Build history of the part. All positions in model axes, mm. Round coordinates to 2 decimals unless told otherwise and drop trailing zeros. Order: outer loops, then holes, each group sorted by start corner. A loop starts at its lowest first (then second) coordinate and runs counter-clockwise, first axis right, second up. Notation, with made-up numbers: M -36,-3 L -31,-3 A21 ccw -31,15 Z; hole C 11.25,-18.5 d6. An arc over 180 degrees is marked long. Use CSV: the item, a comma, the result in double quotes.
from build123d import *

# Parameters (mm, degrees)
SKETCH1_W           = 100
SKETCH1_H           = 120
BOSS_EXTRUDE1_DEPTH = 1.5
SKETCH2_R           = 2.5
CUT_EXTRUDE1_DEPTH  = 1.5
SKETCH4_R           = 2.65
CUT_EXTRUDE2_DEPTH  = 1.5


with BuildPart() as part:
    # Sketch1 → Boss-Extrude1 (new body)
    with BuildSketch(Plane.XY):
        with Locations((50, 60)):
            Rectangle(SKETCH1_W, SKETCH1_H)
    extrude(amount=BOSS_EXTRUDE1_DEPTH)

    # Sketch2 → Cut-Extrude1 (cut)
    with BuildSketch(Plane(origin=(0, 0, 0), x_dir=(-1, 0, 0), z_dir=(0, 0, -1))):
        with Locations((-82.275, 20)):
            Circle(SKETCH2_R)
        with Locations((-17.725, 20)):
            Circle(SKETCH2_R)
        with Locations((-17.725, 100)):
            Circle(SKETCH2_R)
        with Locations((-82.275, 100)):
            Circle(SKETCH2_R)
    extrude(amount=-CUT_EXTRUDE1_DEPTH, mode=Mode.SUBTRACT)

    # Sketch4 → Cut-Extrude2 (cut)
    with BuildSketch(Plane.XY.offset(1.5)):
        with Locations((50, 50)):
            Circle(SKETCH4_R)
        with Locations((50, 70)):
            Circle(SKETCH4_R)
    extrude(amount=-CUT_EXTRUDE2_DEPTH, mode=Mode.SUBTRACT)


solid = part.part
(1) Wall check: line 1 (Y direction, x = 50, z = 1.05); line 2 (Y direction, x = 17, z = 0.4). Give the ranges that are in metal, low to high. Write a range as from..to.
Answer block:
line 1,"y = 0..47.35, 52.65..67.35, 72.65..120"
line 2,"y = 0..17.61, 22.39..97.61, 102.39..120"
(2) Drop a flat-ended pin along its axis: pin 1 (4 mm diameter, centred on x = 17.725, y = 100, fed in from -Z). Give the stop position or say it passes through.
Answer block:
pin 1,"passes through"
(3) Cut at A-A, the plane y = 100. Give the cut face in (x, z) (3 decimals).
Answer block:
outline,"M 0,0 L 15.225,0 L 15.225,1.5 L 0,1.5 Z; M 20.225,0 L 79.775,0 L 79.775,1.5 L 20.225,1.5 Z; M 84.775,0 L 100,0 L 100,1.5 L 84.775,1.5 Z"
(4) Two-plate mould, pull along Y, no slides. Class faces 1 (the face through (49, 61, 1.5)), 2 (the face through (16.381, 22.108, 0.74)): released by +Y, released by -Y, zero draft, split by the parting line, or undercut.
Answer block:
face 1,"zero draft"
face 2,"undercut"
(5) Cut at B-B, the plane y = 50. Give the cut face in (x, z).
Answer block:
outline,"M 0,0 L 47.35,0 L 47.35,1.5 L 0,1.5 Z; M 52.65,0 L 100,0 L 100,1.5 L 52.65,1.5 Z"
